Can you work these out from the model? Positions are in its coordinate system, mm. Coordinates: 2 decimals unless noted, no trailing zeros. Order: outer loops, then holes, each group sorted by start corner. A loop starts at its lowest first (then second) coordinate and runs counter-clockwise, first axis right, second up. Notation, with made-up numbers: M -4,11 L 20,11 A15 ccw 20,38 Z; hole C 81,-18 d7. An arc over 180 degrees is marked long. Answer as a JSON object with one key per item and string values.
from build123d import *

# Parameters (mm, degrees)
ESQUISSE1_W             = 215.9
ESQUISSE1_H             = 152.4
BOSS_EXTRU_1_DEPTH      = 6.35
CONG_1_R                = 12.7
ENL_V_MAT_EXTRU_1_DEPTH = 133.287433266


with BuildPart() as part:
    # Esquisse1 → Boss.-Extru.1 (new body)
    with BuildSketch(Plane(origin=(0, 0, 0), x_dir=(1, 0, 0), z_dir=(0, 1, 0))):
        Rectangle(ESQUISSE1_W, ESQUISSE1_H)
    extrude(amount=BOSS_EXTRU_1_DEPTH)

    # Congé1
    cong_1_edges = [part.edges().sort_by_distance(p)[0] for p in [
        (107.95, 3.175, 76.2),
        (-107.95, 3.175, 76.2),
    ]]
    fillet(cong_1_edges, radius=CONG_1_R)

    # Esquisse2 → Enlèv. mat.-Extru.1 (cut, through all)
    with BuildSketch(Plane(origin=(0, 6.35, 0), x_dir=(1, 0, 0), z_dir=(0, 1, 0))):
        with BuildLine():
            Line((-44.45, 38.1), (44.45, 38.1))
            ThreePointArc((44.45, 38.1), (48.940128061, 36.240128061), (50.8, 31.75))
            Line((50.8, 31.75), (50.8, -57.15))
            ThreePointArc((50.8, -57.15), (48.940128061, -61.640128061), (44.45, -63.5))
            Line((44.45, -63.5), (-44.45, -63.5))
            ThreePointArc((-44.45, -63.5), (-48.940128061, -61.640128061), (-50.8, -57.15))
            Line((-50.8, -57.15), (-50.8, 31.75))
            ThreePointArc((-50.8, 31.75), (-48.940128061, 36.240128061), (-44.45, 38.1))
        make_face()
    extrude(amount=-ENL_V_MAT_EXTRU_1_DEPTH, mode=Mode.SUBTRACT)


solid = part.part
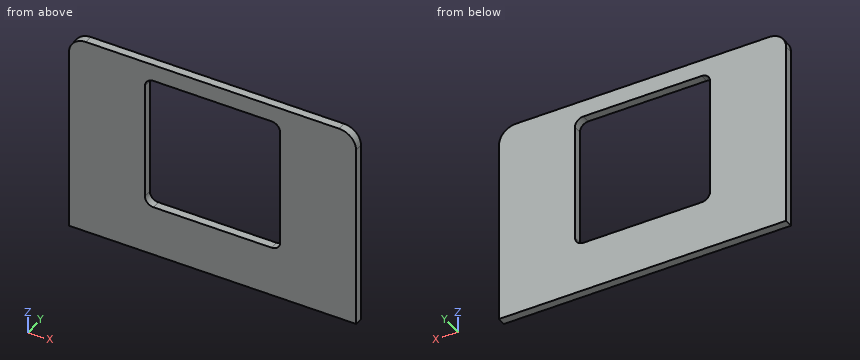
Item 1: I want a section at B-B, the plane z = 8. Write out the boundary of the cut face in (x, y).
Answers follow:
{"outline": "M -107.95,0 L -50.8,0 L -50.8,6.35 L -107.95,6.35 Z; M 50.8,0 L 107.95,0 L 107.95,6.35 L 50.8,6.35 Z"}
Item 2: Please list where these lines run through material, in increasing order: line 1 (Z direction, x = 17, y = 4); line 2 (X direction, y = 1.5, z = 49.5); line 3 (X direction, y = 4, z = -35).
Answers follow:
{"line 1": "z = -76.2 to -38.1, 63.5 to 76.2", "line 2": "x = -107.95 to -50.8, 50.8 to 107.95", "line 3": "x = -107.95 to -49.91, 49.91 to 107.95"}
Item 3: I want a section at C-C, the plane y = 1. Write out the boundary of the cut face in (x, z).
Answers follow:
{"outline": "M -107.95,-76.2 L 107.95,-76.2 L 107.95,63.5 A12.7 ccw 95.25,76.2 L -95.25,76.2 A12.7 ccw -107.95,63.5 Z; hole M -50.8,-31.75 A6.35 ccw -44.45,-38.1 L 44.45,-38.1 A6.35 ccw 50.8,-31.75 L 50.8,57.15 A6.35 ccw 44.45,63.5 L -44.45,63.5 A6.35 ccw -50.8,57.15 Z"}
Item 4: I want a section at A-A, the plane x = -25. Write out the boundary of the cut face in (y, z).
Answers follow:
{"outline": "M 0,-76.2 L 6.35,-76.2 L 6.35,-38.1 L 0,-38.1 Z; M 0,63.5 L 6.35,63.5 L 6.35,76.2 L 0,76.2 Z"}
